Geometry check sheet. Reference: the model listing, model coordinates, mm. Face numbers are marked on the shaded views. Give positions to 0.01 mm unless a question says otherwise; leave off trailing zeros. Order: outer loops, then holes, each group sorted by start corner. A loop starts at its lowest first (then second) coordinate and runs counter-clockwise, first axis right, second up. Notation, with made-up numbers: M -7.75,30.5 L 17.25,30.5 A14 cw 17.25,47.5 Z; hole C 75.25,12 d7. An arc over 180 degrees is marked long. Put each result on its own line as item: value. Start each with the question number.
Q1. Section check C-C on y = -0.8. State how many separate pieces and enclosed holes the cut face has, then the cut area to 3 significant figures.
Q2. Section check B-B on z = -1. Record the cut outline in (x, y).
Q3. Go/stop test with flat-tipped pins: pin 1 (1.5 mm diameter, centred on x = 35.5, y = -0.5, fed in from -Z); pin 2 (0.9 mm diameter, centred on y = 0.5, z = -43, fed in from +X); pin 3 (0.9 mm diameter, centred on y = 0, z = -32, fed in from -X). Record where each tip stops, or that it passes through.
Q4. Material ranges on L1, parallel to X at y = 1.25, z = -14; L2, parallel to X at y = -0.6, z = -36.5; L3, parallel to Z at x = -44.5, y = 0.8, recorded low to high.
Q5. Section check A-A on x = -19. Record the cut outline in (y, z), then the cut area to 3 significant figures.
Q6. Mould release check, pull along Y, two halves, no side actions. Record for the marked faces 1 and 2: +Y half, -Y half, draft (parallel to the pull), parting line (faces both ways), or undercut.
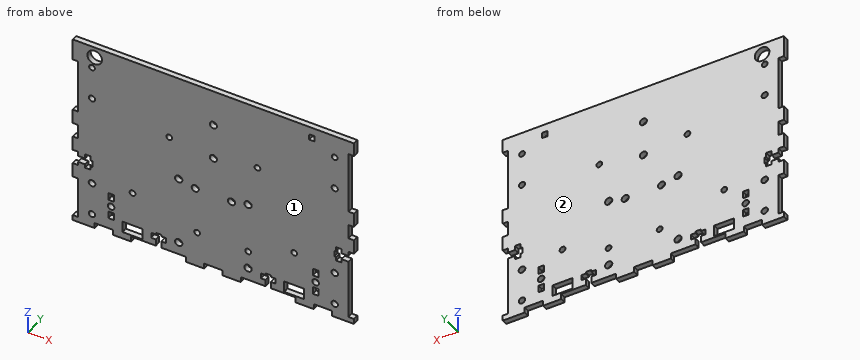
```python
from build123d import *

# Parameters (mm, degrees)
CROQUIS1_R              = 4
SALIENTE_EXTRUIR1_DEPTH = 1.497272789
CROQUIS12_W             = 3
CROQUIS12_H             = 23
CROQUIS12_H_2           = 8
CROQUIS12_H_3           = 18.4
CROQUIS12_H_4           = 9
CORTAR_EXTRUIR10_DEPTH  = 10
CROQUIS13_W             = 3
CROQUIS13_H             = 8
CORTAR_EXTRUIR11_DEPTH  = 10
CROQUIS15_R             = 1.5875
CORTAR_EXTRUIR13_DEPTH  = 10
CROQUIS18_R             = 1.705288108
CROQUIS18_R_2           = 1.572259227
CROQUIS18_R_3           = 1.751719864
CROQUIS18_R_4           = 1.822918829
CORTAR_EXTRUIR15_DEPTH  = 10
CROQUIS19_R             = 1.8
CROQUIS19_W             = 3
CROQUIS19_H             = 4
CORTAR_EXTRUIR16_DEPTH  = 10
CROQUIS20_R             = 1.600000002
CROQUIS20_W             = 10.939065956
CROQUIS20_H             = 6.243980126
CORTAR_EXTRUIR17_DEPTH  = 10
CROQUIS21_R             = 1.951923789
CROQUIS21_R_2           = 2
CORTAR_EXTRUIR18_DEPTH  = 10
CROQUIS22_R             = 1.951923789
CORTAR_EXTRUIR19_DEPTH  = 10


with BuildPart() as part:
    # Croquis1 → Saliente-Extruir1 (new, symmetric)
    with BuildSketch(Plane(origin=(0, 0, 0), x_dir=(1, 0, 0), z_dir=(0, 1, 0))):
        Polygon((-77, -42), (-77, -54), (77, -54), (77, -42), (74, -42), (74, -28), (77, -28), (77, -20), (74, -20), (74, -12), (77, -12), (77, -4), (74, -4), (74, -1.5), (74, 1.5), (74, 4), (77, 4), (77, 12), (74, 12), (74, 14.497912952), (70.25, 14.497912952), (70.25, 12), (67.25, 12), (67.25, 14.497912952), (66.27, 14.497912952), (66.27, 17.992083938), (67.25, 17.992083938), (67.25, 20), (70.25, 20), (70.25, 17.992083938), (74, 17.992083938), (74, 20), (77, 20), (77, 28), (74, 28), (74, 42), (77, 42), (77, 54), (65, 54), (65, 51), (55, 51), (55, 54), (45, 54), (45, 51), (31.5, 51), (31.5, 47.25), (34, 47.25), (34, 44.25), (31.5, 44.25), (31.5, 43.27), (28.5, 43.27), (28.5, 44.25), (26, 44.25), (26, 47.25), (28.5, 47.25), (28.5, 51), (15, 51), (15, 54), (5, 54), (5, 51), (-5, 51), (-5, 54), (-15, 54), (-15, 51), (-28.5, 51), (-28.5, 47.25), (-26, 47.25), (-26, 44.25), (-28.5, 44.25), (-28.5, 43.27), (-31.5, 43.27), (-31.5, 44.25), (-34, 44.25), (-34, 47.25), (-31.5, 47.25), (-31.5, 51), (-45, 51), (-45, 54), (-55, 54), (-55, 51), (-65, 51), (-65, 54), (-77, 54), (-77, 42), (-74, 42), (-74, 28), (-77, 28), (-77, 20), (-74, 20), (-74, 17.992083938), (-70.25, 17.992083938), (-70.25, 20), (-67.25, 20), (-67.25, 17.992083938), (-66.27, 17.992083938), (-66.27, 14.497912952), (-67.25, 14.497912952), (-67.25, 12), (-70.25, 12), (-70.25, 14.497912952), (-74, 14.497912952), (-74, 12), (-77, 12), (-77, 4), (-74, 4), (-74, 1.5), (-74, -1.5), (-74, -4), (-77, -4), (-77, -12), (-74, -12), (-74, -20), (-77, -20), (-77, -28), (-74, -28), (-74, -42), align=None)
        with Locations(Location((-65, -48, 0), (0, 0, 270))):
            Circle(CROQUIS1_R, mode=Mode.SUBTRACT)
        with BuildLine():
            Line((55, -49.6), (53, -49.6))
            ThreePointArc((53, -49.6), (52.646446609, -49.453553391), (52.5, -49.1))
            Line((52.5, -49.1), (52.5, -46.4))
            Line((52.5, -46.4), (55.5, -46.4))
            Line((55.5, -46.4), (55.5, -49.1))
            ThreePointArc((55.5, -49.1), (55.353553391, -49.453553391), (55, -49.6))
        make_face(mode=Mode.SUBTRACT)
    extrude(amount=SALIENTE_EXTRUIR1_DEPTH, both=True)

    # Croquis12 → Cortar-Extruir10 (cut)
    with BuildSketch(Plane.XZ.offset(1.497272789)):
        with Locations((-75.5, -39.5)):
            Rectangle(CROQUIS12_W, CROQUIS12_H)
        with Locations((-75.5, 24)):
            Rectangle(CROQUIS12_W, CROQUIS12_H_2)
        with Locations((75.5, -24)):
            Rectangle(CROQUIS12_W, CROQUIS12_H_2)
        with Locations((75.5, 37.2)):
            Rectangle(CROQUIS12_W, CROQUIS12_H_3)
        with Locations((75.5, -46.5)):
            Rectangle(CROQUIS12_W, CROQUIS12_H_4)
    extrude(amount=-CORTAR_EXTRUIR10_DEPTH, mode=Mode.SUBTRACT)

    # Croquis13 → Cortar-Extruir11 (cut)
    with BuildSketch(Plane.XZ.offset(1.497272789)):
        with Locations((75.5, 24)):
            Rectangle(CROQUIS13_W, CROQUIS13_H)
    extrude(amount=-CORTAR_EXTRUIR11_DEPTH, mode=Mode.SUBTRACT)

    # Croquis15 → Cortar-Extruir13 (cut)
    with BuildSketch(Plane(origin=(0, 1.497272789, 0), x_dir=(1, 0, 0), z_dir=(0, 1, 0))):
        with Locations(Location((-8.89, 34.036119394, 0), (0, 0, 270))):
            Circle(CROQUIS15_R)
        with Locations(Location((19.05, 34.036119394, 0), (0, 0, 270))):
            Circle(CROQUIS15_R)
        with Locations(Location((24.13, -18.033880606, 0), (0, 0, 270))):
            Circle(CROQUIS15_R)
        with Locations(Location((-24.13, -16.763880606, 0), (0, 0, 270))):
            Circle(CROQUIS15_R)
    extrude(amount=-CORTAR_EXTRUIR13_DEPTH, mode=Mode.SUBTRACT)

    # Croquis18 → Cortar-Extruir15 (cut)
    with BuildSketch(Plane(origin=(0, 1.497272789, 0), x_dir=(1, 0, 0), z_dir=(0, 1, 0))):
        with Locations(Location((66.447956343, -22.895683893, 0), (0, 0, 270))):
            Circle(CROQUIS18_R)
        with Locations(Location((66.447956343, -41.396232491, 0), (0, 0, 270))):
            Circle(CROQUIS18_R_2)
        with Locations(Location((66.447956343, 46.216518088, 0), (0, 0, 270))):
            Circle(CROQUIS18_R_3)
        with Locations(Location((66.447956343, 27.741721108, 0), (0, 0, 270))):
            Circle(CROQUIS18_R_4)
        with Locations(Location((-66.447956343, 27.741721108, 0), (0, 0, 270))):
            Circle(CROQUIS18_R_4)
        with Locations(Location((-66.447956343, 46.216518088, 0), (0, 0, 270))):
            Circle(CROQUIS18_R_3)
        with Locations(Location((-66.447956343, -41.396232491, 0), (0, 0, 270))):
            Circle(CROQUIS18_R_2)
        with Locations(Location((-66.447956343, -22.895683893, 0), (0, 0, 270))):
            Circle(CROQUIS18_R)
    extrude(amount=-CORTAR_EXTRUIR15_DEPTH, mode=Mode.SUBTRACT)

    # Croquis19 → Cortar-Extruir16 (cut)
    with BuildSketch(Plane(origin=(0, 1.497272789, 0), x_dir=(1, 0, 0), z_dir=(0, 1, 0))):
        with Locations(Location((-56, 37.5, 0), (0, 0, 270))):
            Circle(CROQUIS19_R)
        with Locations(Location((56, 37.5, 0), (0, 0, 270))):
            Circle(CROQUIS19_R)
        with Locations((-56, 32)):
            Rectangle(CROQUIS19_W, CROQUIS19_H)
        with Locations((-56, 43)):
            Rectangle(CROQUIS19_W, CROQUIS19_H)
        with Locations((56, 43)):
            Rectangle(CROQUIS19_W, CROQUIS19_H)
        with Locations((56, 32)):
            Rectangle(CROQUIS19_W, CROQUIS19_H)
    extrude(amount=-CORTAR_EXTRUIR16_DEPTH, mode=Mode.SUBTRACT)

    # Croquis20 → Cortar-Extruir17 (cut)
    with BuildSketch(Plane(origin=(0, 1.497272789, 0), x_dir=(1, 0, 0), z_dir=(0, 1, 0))):
        with Locations(Location((-44.25, 24.7, 0), (0, 0, 270))):
            Circle(CROQUIS20_R)
        with Locations((-44.267144923, 47.081261314)):
            Rectangle(CROQUIS20_W, CROQUIS20_H)
    cortar_extruir17 = extrude(amount=-CORTAR_EXTRUIR17_DEPTH, mode=Mode.SUBTRACT)

    # Simetría1: Cortar-Extruir17 across plane
    add(cortar_extruir17.mirror(Plane(origin=(0, 0, 0), x_dir=(0, 0, 1), z_dir=(1, 0, 0))), mode=Mode.SUBTRACT)

    # Croquis21 → Cortar-Extruir18 (cut)
    with BuildSketch(Plane(origin=(0, 1.497272789, 0), x_dir=(1, 0, 0), z_dir=(0, 1, 0))):
        with Locations(Location((0, -33.825, 0), (0, 0, 270))):
            Circle(CROQUIS21_R)
        with Locations(Location((0, -13.975, 0), (0, 0, 270))):
            Circle(CROQUIS21_R)
        with Locations(Location((19, 6.05, 0), (0, 0, 270))):
            Circle(CROQUIS21_R_2)
        with Locations(Location((19, 44.05, 0), (0, 0, 270))):
            Circle(CROQUIS21_R_2)
        with Locations(Location((-19, 44.05, 0), (0, 0, 270))):
            Circle(CROQUIS21_R_2)
        with Locations(Location((-19, 6.05, 0), (0, 0, 270))):
            Circle(CROQUIS21_R_2)
    extrude(amount=-CORTAR_EXTRUIR18_DEPTH, mode=Mode.SUBTRACT)

    # Croquis22 → Cortar-Extruir19 (cut)
    with BuildSketch(Plane(origin=(0, 1.497272789, 0), x_dir=(1, 0, 0), z_dir=(0, 1, 0))):
        with Locations(Location((-9.925, 8, 0), (0, 0, 270))):
            Circle(CROQUIS22_R)
        with Locations(Location((9.925, 8, 0), (0, 0, 270))):
            Circle(CROQUIS22_R)
    extrude(amount=-CORTAR_EXTRUIR19_DEPTH, mode=Mode.SUBTRACT)


solid = part.part
```
Results found:
1. separate pieces: 1
1. enclosed holes: 32
1. area: 15,300 mm^2
2. outline: M -74,-1.5 L 74,-1.5 L 74,1.5 L -74,1.5 Z
3. pin 1: stops at z = -51
3. pin 2: stops at x = 74
3. pin 3: stops at x = -74
4. L1: x = -74 to -70.25, -67.25 to 67.25, 70.25 to 74
4. L2: x = -74 to -57.5, -54.5 to 54.5, 57.5 to 74
4. L3: z = -51 to -50.2, -43.96 to -26.28, -23.12 to 54
5. outline: M -1.5,-51 L 1.5,-51 L 1.5,-46.05 L -1.5,-46.05 Z; M -1.5,-42.05 L 1.5,-42.05 L 1.5,-8.05 L -1.5,-8.05 Z; M -1.5,-4.05 L 1.5,-4.05 L 1.5,54 L -1.5,54 Z
5. area: 290 mm^2
6. face 1: -Y half
6. face 2: +Y half
